```python
from build123d import *

# Parameters (mm, degrees)
SCREW_HOLES_COUNT = 12


with BuildPart() as part:
    # Cross Section → Main (revolve)
    with BuildSketch(Plane.XY):
        Polygon((-38.1, 0), (-38.1, -3.175), (-39.624, -3.175), (-39.624, -15.875), (-40.005, -15.215088642), (-40.005, -3.175), (-46.863, -3.175), (-46.863, 9.525), (-44.45, 9.525), (-44.45, 0), align=None)
    revolve(axis=Axis((0, 55, 0), (0, -1, 0)))

    # Sketch7 → #0-80 Tapped Hole1 (revolve, cut)
    with BuildSketch(Plane(origin=(-41.275, 0, 0), x_dir=(0, 0, 1), z_dir=(1, 0, 0))):
        Polygon((0, 0), (0, 3.532890611), (0.59563, 3.175), (0.59563, 0), align=None)
    f_0_80_tapped_hole1 = revolve(axis=Axis((-41.275, 6.35, 0), (0, -1, 0)), mode=Mode.SUBTRACT)

    # Screw Holes: #0-80 Tapped Hole1 ×12 about axis
    screw_holes_axis = Axis((0, 0, 0), (0, 1, 0))
    for i in range(1, SCREW_HOLES_COUNT):
        add(f_0_80_tapped_hole1.rotate(screw_holes_axis, i * 360 / SCREW_HOLES_COUNT), mode=Mode.SUBTRACT)


solid = part.part
```
Can you work these out from the model? Positions are in its coordinate system, mm. A direction names the side the tool comes from. Give positions to 0.01 mm unless a question says otherwise; leave off trailing zeros. Write each loop counter-clockwise with the first axis right and the second up, starting at its lowest first coordinate (ties: lowest second). Pieces come first, ordered by that corner, then holes. Notation, with made-up numbers: (59, -5.5) -> (91, -5.5) arc R31 ccw to (91, 22.5) -> close; hole circle Ø9 at (87, -16). An arc over 180 degrees is marked (long way). Write item = value, one per line.
(1) Suppose I cut it at B-B on y = -12.75. Write out the boundary of the cut face in (x, z) (3 decimals), then the cut area to 3 significant figures.
Worked out:
outline = circle Ø80.01 at (0, 0); hole circle Ø79.248 at (0, 0)
area = 95.3 mm^2
(2) Thinking about a two-plate mould opening in Z: for faces 1 (the face through (-42.397, 4.696, -13.352)), 2 (the face through (37.2, 3.3, 28.5)), 3 (the face through (-21, -3.175, -32)), 4 (the face through (-28, 9.525, -35)), which applies, released by +Z, released by -Z, zero draft, split by the parting line, or undercut?
Worked out:
face_1 = undercut
face_2 = split by the parting line
face_3 = undercut
face_4 = zero draft
(3) For faces 5 (the face through (30.235, -1.61, 23.183)), 6 (the face through (-33, 0, -20)), 7 (the face through (-38.158, -9.111, -12.016)), which set-ups out of +Z, -Z, +X, -X, +Y, -Y let a thin tool reach every point of the face, with its end or its side?
Worked out:
face_5 = +Y, -Y
face_6 = +Y
face_7 = -Y
(4) I'm going to push flat-ended pins straight in: P1, Ø1.9, axis at x = -20.64, z = 35.75, coming from the +Y side; P2, Ø1.4, axis at x = 20.64, z = 35.75, coming from the -Y side (3 decimals); P3, Ø5, axis at y = -6.5, z = -19.5, coming from the +X side; P4, Ø24, axis at x = 14, z = -13.5, coming from the -Y side. Where does each tip first touch, or does it pass through?
Worked out:
P1 = 0
P2 = -3.175
P3 = 36.21
P4 = through
(5) I need wall thicknesses on probe 1 along Z at (x, y) = (0, -1.9); probe 2 along X at (y, z) = (5.25, 0). Which ranges of each line are inside material? Lowest first, please. Write a range as from..to.
Worked out:
probe_1 = -46.86..-41.87, -40.68..-38.1, 38.1..40.68, 41.87..46.86
probe_2 = -46.86..-44.45, 44.45..46.86
(6) Suppose I cut it at A-A on y = 4.75. Write out the boundary of the cut face in (x, z), then the cut area to 3 significant figures.
Worked out:
outline = circle Ø93.73 at (0, 0); hole circle Ø88.9 at (0, 0)
area = 692 mm^2
